Autodesk Inventor part; units mm, degrees
ref_plane "YZ Plane" through (0, 0, 0) normal (1, 0, 0) x (0, 1, 0)
ref_plane "XZ Plane" through (0, 0, 0) normal (0, 1, 0) x (-1, 0, 0)
ref_plane "XY Plane" through (0, 0, 0) normal (0, 0, 1) x (1, 0, 0)
sketch "Sketch1" plane through (0, 0, 0) normal (0, 0, 1) x (1, 0, 0)
  line L0 (7.598, 5.174) -> (-5.174, 7.598)
  line L1 (5.174, -7.598) -> (7.598, 5.174)
  line L2 (-7.598, -5.174) -> (5.174, -7.598)
  line L3 (-5.174, 7.598) -> (-7.598, -5.174)
  line L4 (-11.1048, -7.562) -> (-7.562, 11.1048)
  line L5 (-7.562, 11.1048) -> (11.1048, 7.562)
  line L6 (11.1048, 7.562) -> (7.562, -11.1048)
  line L7 (7.562, -11.1048) -> (-11.1048, -7.562)
  point P0 (0, 0)
  dimension "d0" = 3
  dimension "d1" = 3
  dimension "d2" = 3
  dimension "d3" = 3
ref_plane "Work Plane1" through (0, 0, -5) normal (0, 0, 1) x (1, 0, 0)
sketch "Sketch2" plane through (0, 0, -5) normal (0, 0, 1) x (1, 0, 0)
  line L0 (7.598, 5.174) -> (-5.174, 7.598)
  line L1 (-7.562, 11.1048) -> (11.1048, 7.562)
  line L2 (-11.1048, -7.562) -> (-7.562, 11.1048)
  line L3 (7.562, -11.1048) -> (-11.1048, -7.562)
  line L4 (11.1048, 7.562) -> (7.562, -11.1048)
  line L5 (5.174, -7.598) -> (7.598, 5.174)
  line L6 (-7.598, -5.174) -> (5.174, -7.598)
  line L7 (-5.174, 7.598) -> (-7.598, -5.174)
  point P0 (0, 0)
extrude "Extrusion1" add sketch "Sketch2" against normal blind 92
sketch "Sketch3" plane through (0, 0, -5) normal (0, 0, 1) x (1, 0, 0)
  line L0 (-11.1048, -7.562) -> (7.562, -11.1048)
  line L1 (7.562, -11.1048) -> (11.1048, 7.562)
  line L2 (11.1048, 7.562) -> (-7.562, 11.1048)
  line L3 (-7.562, 11.1048) -> (-11.1048, -7.562)
  line L4 (7.598, 5.174) -> (5.174, -7.598)
  line L5 (5.174, -7.598) -> (-7.598, -5.174)
  line L6 (-7.598, -5.174) -> (-5.174, 7.598)
  line L7 (-5.174, 7.598) -> (7.598, 5.174)
  circle A0 centre (0, 0) radius 1.5
  dimension "d6" = 3
extrude "Extrusion2" add sketch "Sketch3" along normal blind 3 contours L3 L2 L1 L0 | L4 L5 L6 L7
properties part number "Casing"
Work out the finished part from the listing and answer in its coordinate system (mm). A direction names the side the tool comes from. Coordinates: 2 decimals unless noted, no trailing zeros. Order: outer loops, then holes, each group sorted by start corner. A loop starts at its lowest first (then second) coordinate and runs counter-clockwise, first axis right, second up. Notation, with made-up numbers: M 4.5,-10.5 L 39.5,-10.5 A22 ccw 39.5,15.5 Z; hole C 64.5,70 d2. An arc over 180 degrees is marked long. Use CSV: the item, a comma, the result in double quotes.
1) Flat-ended cylindrical pins translate along their axes: pin 1 Ø2 at (x, z) = (-3.5, -29) entering from +Y; pin 2 Ø5 at (y, z) = (7, -24) entering from -X; pin 3 Ø1 at (y, z) = (-6.5, -44.5) entering from +X. Find the tip coordinate at first contact, or state that the pin passes through.
Worked out:
pin 1,"stops at y = 10.52"
pin 2,"stops at x = -8.82"
pin 3,"stops at x = 8.53"
2) Consider line 1 (Z direction, x = -1.75, y = -4.75); line 2 (X direction, y = -4.75, z = -34); line 3 (Y direction, x = 0, z = -3.05). Determine where each line is inside the solid, lowest interval first. Write a range as [from, to].
Worked out:
line 1,"z = [-5, -2]"
line 2,"x = [-10.57, -7.52], [5.71, 8.77]"
line 3,"y = [-9.67, -1.5], [1.5, 9.67]"
3) Determine the mould class of faces 3 (the face through (9.36, -1.64, -48.84)), 4 (the face through (-9.36, 1.64, -48.84)), 5 (the face through (-1.5, -0.07, -3.52)), 6 (the face through (-8, 0, -97)) for opening direction Y: released by +Y, released by -Y, zero draft, split by the parting line, or undercut.
Worked out:
face 3,"released by -Y"
face 4,"released by +Y"
face 5,"undercut"
face 6,"zero draft"
4) For faces 1 (the face through (-1.3, -6.37, -50.36)), 2 (the face through (1.64, 9.36, -48.84)), determine the directions among +Z, -Z, +X, -X, +Y, -Y from which every point of the face is accessible in a straight line to the end or side of a thin tool.
Worked out:
face 1,"-Z"
face 2,"+Z, -Z, +X, +Y"
5) Section A-A on x = 0.5 is taken. Write down the section's boundary in (y, z).
Worked out:
outline,"M -9.76,-97 L -6.71,-97 L -6.71,-5 L -1.41,-5 L -1.41,-2 L -9.76,-2 Z; M 1.41,-5 L 6.52,-5 L 6.52,-97 L 9.57,-97 L 9.57,-2 L 1.41,-2 Z"
6) Section D-D on y = 6 is taken. Write down the section's boundary in (x, z), plus the area to 3 significant figures.
Worked out:
outline,"M -8.53,-97 L -5.48,-97 L -5.48,-5 L 3.25,-5 L 3.25,-97 L 10.81,-97 L 10.81,-2 L -8.53,-2 Z"
area,"1,030 mm^2"
7) Section C-C on y = 0 is taken. Write down the section's boundary in (x, z).
Worked out:
outline,"M -9.67,-97 L -6.62,-97 L -6.62,-5 L -1.5,-5 L -1.5,-2 L -9.67,-2 Z; M 1.5,-5 L 6.62,-5 L 6.62,-97 L 9.67,-97 L 9.67,-2 L 1.5,-2 Z"
8) Section B-B on z = -67.5 is taken. Write down the section's boundary in (x, y).
Worked out:
outline,"M -11.1,-7.56 L 7.56,-11.1 L 11.1,7.56 L -7.56,11.1 Z; hole M -7.6,-5.17 L 5.17,-7.6 L 7.6,5.17 L -5.17,7.6 Z"
